The listing builds one solid part. Answer for the finished solid, in the listing's coordinates (mm). Round coordinates to 2 decimals unless told otherwise and drop trailing zeros. Put each result on its own line as item: value. Start each with the question number.
1. Consider line 1 (Z direction, x = 12.7, y = -0.6) (3 decimals); line 2 (Z direction, x = -12, y = -0.7) (3 decimals); line 3 (X direction, y = -1.05, z = -6). Determine where each line is inside the solid, lowest interval first.
2. The part is cut by section A-A (y = -0.5). Count the separate pieces of the cut face and the enclosed holes in it, then the cut area to 3 significant figures.
3. This flat-tipped pin is pushed along its axis until it touches: pin 1 Ø4 at (x, z) = (12.7, 0) entering from +Y. Where does it stop, or does it pass through?
from build123d import *

# Parameters (mm, degrees)
F0_R     = 2.15265
F1_DEPTH = 1.5875


with BuildPart() as f1:
    # F0 (on Front) → F1 (new body)
    with BuildSketch(Plane.XZ):
        with BuildLine():
            Line((146.05, 9.525), (-146.05, 9.525))
            ThreePointArc((-146.05, 9.525), (-150.540128, 7.665128), (-152.4, 3.175))
            Line((-152.4, 3.175), (-152.4, -3.175))
            ThreePointArc((-152.4, -3.175), (-150.540128, -7.665128), (-146.05, -9.525))
            Line((-146.05, -9.525), (-82.55, -9.525))
            Line((-82.55, -9.525), (-19.05, -9.525))
            Line((-19.05, -9.525), (146.05, -9.525))
            ThreePointArc((146.05, -9.525), (150.540128, -7.665128), (152.4, -3.175))
            Line((152.4, -3.175), (152.4, 3.175))
            ThreePointArc((152.4, 3.175), (150.540128, 7.665128), (146.05, 9.525))
        make_face()
        with Locations((-139.7, 0)):
            Circle(F0_R, mode=Mode.SUBTRACT)
        with Locations((-114.3, 0)):
            Circle(F0_R, mode=Mode.SUBTRACT)
        with Locations((-76.2, 0)):
            Circle(F0_R, mode=Mode.SUBTRACT)
        with Locations((-50.8, 0)):
            Circle(F0_R, mode=Mode.SUBTRACT)
        with Locations((-12.7, 0)):
            Circle(F0_R, mode=Mode.SUBTRACT)
        with Locations((12.7, 0)):
            Circle(F0_R, mode=Mode.SUBTRACT)
        with Locations((50.8, 0)):
            Circle(F0_R, mode=Mode.SUBTRACT)
        with Locations((76.2, 0)):
            Circle(F0_R, mode=Mode.SUBTRACT)
        with Locations((114.3, 0)):
            Circle(F0_R, mode=Mode.SUBTRACT)
        with Locations((139.7, 0)):
            Circle(F0_R, mode=Mode.SUBTRACT)
    extrude(amount=F1_DEPTH)


solid = f1.part
Resolved:
1. line 1: -9.525 to -2.153, 2.153 to 9.525
1. line 2: -9.525 to -2.036, 2.036 to 9.525
1. line 3: -151.74 to 151.74
2. separate pieces: 1
2. enclosed holes: 10
2. area: 5,630 mm2
3. pin 1: through
